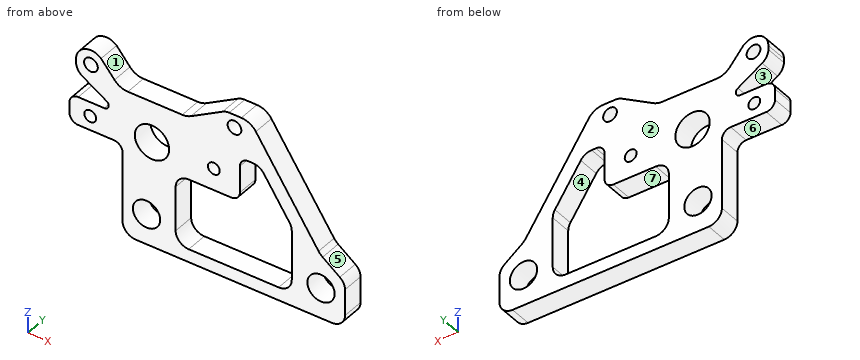
```python
from build123d import *

# Parameters (mm, degrees)
SKETCH4_R           = 2
SKETCH4_R_2         = 1.7272
SKETCH4_R_3         = 5
SKETCH4_R_4         = 3.96875
BOSS_EXTRUDE2_DEPTH = 6.35
FILLET1_R           = 5.08
FILLET7_R           = 3.81
FILLET9_R           = 5.08
FILLET10_R          = 1.27
FILLET11_R          = 3.81
FILLET12_R          = 2.54
FILLET13_R          = 3.81


with BuildPart() as part:
    # Sketch4 → Boss-Extrude2 (new body)
    with BuildSketch(Plane(origin=(0, 0, 0), x_dir=(1, 0, 0), z_dir=(0, 1, 0))):
        with BuildLine():
            Line((22.483900583, -18.4375), (28.735494078, -18.4375))
            Line((28.735494078, -18.4375), (48.985566477, 12.027918285))
            Line((48.985566477, 12.027918285), (54.680415238, 16.319294633))
            ThreePointArc((54.680415238, 16.319294633), (55.797199918, 17.662082259), (56.1975, 19.362095927))
            Line((56.1975, 19.362095927), (56.1975, 26.9875))
            ThreePointArc((56.1975, 26.9875), (55.081576836, 29.681576836), (52.3875, 30.7975))
            Line((52.3875, 30.7975), (-4.7625, 30.7975))
            ThreePointArc((-4.7625, 30.7975), (-7.456576836, 29.681576836), (-8.5725, 26.9875))
            Line((-8.5725, 26.9875), (-8.5725, 12.607500122))
            Line((-8.5725, 12.607500122), (-8.5725, 4.1275))
            Line((-8.5725, 4.1275), (-24.03032317, 4.1275))
            Line((-24.03032317, 4.1275), (-24.03032317, -4.1275))
            Line((-24.03032317, -4.1275), (-9.399713355, -4.1275))
            Line((-9.399713355, -4.1275), (-22.098, -11.933490986))
            Line((-22.098, -11.933490986), (-22.098, -15.24))
            ThreePointArc((-22.098, -15.24), (-19.494143335, -19.203185162), (-14.822948297, -18.386580561))
            Line((-14.822948297, -18.386580561), (-9.399713355, -11.933490986))
            Line((-9.399713355, -11.933490986), (10.16293305, -11.933490986))
            Line((10.16293305, -11.933490986), (20.583679925, -17.929811531))
            ThreePointArc((20.583679925, -17.929811531), (21.500464498, -18.308390309), (22.483900583, -18.4375))
        make_face()
        with Locations((-17.78, -15.24)):
            Circle(SKETCH4_R, mode=Mode.SUBTRACT)
        with Locations((-18.000000004, 0)):
            Circle(SKETCH4_R_2, mode=Mode.SUBTRACT)
        Circle(SKETCH4_R_3, mode=Mode.SUBTRACT)
        with Locations((24.012521227, -14.703599027)):
            Circle(SKETCH4_R, mode=Mode.SUBTRACT)
        with Locations((18.000000004, 0)):
            Circle(SKETCH4_R_2, mode=Mode.SUBTRACT)
        with Locations((-1.5875, 21.9075)):
            Circle(SKETCH4_R_4, mode=Mode.SUBTRACT)
        Polygon((6.882386285, 6.3725), (6.882386285, 26.9875), (40.692955064, 26.9875), (40.692955064, 7.472580753), (31.404651622, -6.501297657), (25.585775375, -6.501297657), (25.585775375, 6.3725), align=None, mode=Mode.SUBTRACT)
        with Locations((49.2125, 21.9075)):
            Circle(SKETCH4_R_4, mode=Mode.SUBTRACT)
    extrude(amount=-BOSS_EXTRUDE2_DEPTH)

    # Fillet1
    fillet1_edges = [part.edges().sort_by_distance(p)[0] for p in [
        (48.985566477, -3.175, -12.027918285),
        (28.735494078, -3.175, 18.4375),
    ]]
    fillet(fillet1_edges, radius=FILLET1_R)

    # Fillet7
    fillet7_edges = [part.edges().sort_by_distance(p)[0] for p in [
        (40.692955064, -3.175, -7.472580753),
        (40.692955064, -3.175, -26.9875),
        (6.882386285, -3.175, -26.9875),
        (6.882386285, -3.175, -6.3725),
    ]]
    fillet(fillet7_edges, radius=FILLET7_R)

    # Fillet9
    fillet9_edges = [part.edges().sort_by_distance(p)[0] for p in [
        (10.16293305, -3.175, 11.933490986),
        (-9.399713355, -3.175, 11.933490986),
    ]]
    fillet(fillet9_edges, radius=FILLET9_R)

    # Fillet10
    fillet10_edges = [part.edges().sort_by_distance(p)[0] for p in [
        (-9.399713355, -3.175, 4.1275),
    ]]
    fillet(fillet10_edges, radius=FILLET10_R)

    # Fillet11
    fillet11_edges = [part.edges().sort_by_distance(p)[0] for p in [
        (-22.098, -3.175, 11.933490986),
    ]]
    fillet(fillet11_edges, radius=FILLET11_R)

    # Fillet12
    fillet12_edges = [part.edges().sort_by_distance(p)[0] for p in [
        (25.585775375, -3.175, -6.3725),
        (25.585775375, -3.175, 6.501297657),
        (-24.03032317, -3.175, 4.1275),
        (-24.03032317, -3.175, -4.1275),
        (-8.5725, -3.175, -4.1275),
    ]]
    fillet(fillet12_edges, radius=FILLET12_R)

    # Fillet13
    fillet13_edges = [part.edges().sort_by_distance(p)[0] for p in [
        (31.404651622, -3.175, 6.501297657),
    ]]
    fillet(fillet13_edges, radius=FILLET13_R)


solid = part.part
```
Input: part model. Units: mm. Frame: model coordinates. Face numbers are marked on the shaded views. A direction names the side the tool comes from. Give positions to 0.01 mm unless a question says otherwise; leave off trailing zeros. Write each loop counter-clockwise with the first axis right and the second up, starting at its lowest first coordinate (ties: lowest second). Pieces come first, ordered by that corner, then holes. Notation, with made-up numbers: (38, 22.5) - (67, 22.5) arc R10 ccw to (67, 27.5) - close; hole circle Ø1 at (4, -30.5). An arc over 180 degrees is marked (long way). Write item = value, one per line. Start each with the question number.
1. Section query C-C, the plane x = -17.78. Output: boundary loops of the cut face in (y, z), then the cut area to 3 significant figures.
2. Access query for the marked faces 1, 2, 3 and 4. Directions: +Z, -Z, +X, -X, +Y, -Y. A direction counts if a zero-diameter tool reaches every point of the face in a straight line with its end or side. Return the directions, or none.
3. Section query A-A, the plane x = 0. Output: boundary loops of the cut face in (y, z), then the cut area to 3 significant figures.
4. Ray query, L1, parallel to X at y = -3.75, z = 17; L2, parallel to X at y = -3.25, z = -23; L3, parallel to X at y = -3.5, z = 14. Return the intervals inside material, ascending.
5. First-contact query: pin 1 Ø1 at (y, z) = (-2.5, 7) entering from -X; pin 2 Ø3 at (x, y) = (-18, -2.5) entering from -Z; pin 3 Ø2.5 at (x, z) = (24.01, 14.7) entering from +Y; pin 4 Ø3 at (x, y) = (-19.5, -3.5) entering from +Z. Flat tips, straight axial feed; report the tip coordinate or a pass-through.
6. Section query B-B, the plane z = -15. Output: boundary loops of the cut face in (x, y), then the cut area to 3 significant figures.
7. Section query D-D, the plane z = 0. Output: boundary loops of the cut face in (x, y).
8. Mould query, pull axis X, two halves, no side actions, for the marked faces 5, 6 and 7. Classes: released by +X, released by -X, zero draft, split by the parting line, or undercut.
Check sheet entries:
q1.outline = (-6.35, -4.13) - (0, -4.13) - (0, -1.71) - (-6.35, -1.71) - close; (-6.35, 1.71) - (0, 1.71) - (0, 4.13) - (-6.35, 4.13) - close; (-6.35, 9.28) - (0, 9.28) - (0, 13.24) - (-6.35, 13.24) - close; (-6.35, 17.24) - (0, 17.24) - (0, 19.56) - (-6.35, 19.56) - close
q1.area = 70.5 mm2
q2.face_1 = +Z, +Y, -Y
q2.face_2 = +Z, -Z, +X, -X, +Y
q2.face_3 = -X, +Y, -Y
q2.face_4 = +Y, -Y
q3.outline = (-6.35, -30.8) - (0, -30.8) - (0, -25.54) - (-6.35, -25.54) - close; (-6.35, -18.27) - (0, -18.27) - (0, -5) - (-6.35, -5) - close; (-6.35, 5) - (0, 5) - (0, 11.93) - (-6.35, 11.93) - close
q3.area = 162 mm2
q4.L1 = -21.72 to -18.73, -16.83 to -13.66, 18.97 to 29.55
q4.L2 = -8.57 to -5.4, 2.23 to 6.88, 40.69 to 45.4, 53.03 to 56.2
q4.L3 = -22.1 to -19.35, -16.21 to -11.14, 13.75 to 22.14, 25.88 to 31.69
q5.pin_1 = -14.89
q5.pin_2 = -4.13
q5.pin_3 = through
q5.pin_4 = 19.55
q6.outline = (-8.57, -6.35) - (6.88, -6.35) - (6.88, 0) - (-8.57, 0) - close; (40.69, -6.35) - (52.93, -6.35) - (52.93, 0) - (40.69, 0) - close
q6.area = 176 mm2
q7.outline = (-24.03, -6.35) - (-19.73, -6.35) - (-19.73, 0) - (-24.03, 0) - close; (-16.27, -6.35) - (-5, -6.35) - (-5, 0) - (-16.27, 0) - close; (5, -6.35) - (16.27, -6.35) - (16.27, 0) - (5, 0) - close; (19.73, -6.35) - (25.59, -6.35) - (25.59, 0) - (19.73, 0) - close; (35.73, -6.35) - (40.99, -6.35) - (40.99, 0) - (35.73, 0) - close
q8.face_5 = released by +X
q8.face_6 = zero draft
q8.face_7 = undercut
